```python
from build123d import *

# Parameters (mm, degrees)
F1_DEPTH = 36
F2_R     = 15
F3_T     = -2.5
F4_W     = 67
F4_H     = 27
F5_DEPTH = 3
F6_DEPTH = 100
F7_DEPTH = 5


with BuildPart() as f1:
    # F0 (on Right) → F1 (new body, symmetric)
    with BuildSketch(Plane.YZ):
        Polygon((-28, 0), (0, 0), (0, 32), (-60, 32), (-60, 0), (-60, -28), (-28, -28), align=None)
    extrude(amount=F1_DEPTH, both=True)

    # F2
    f2_edges = [f1.edges().sort_by_distance(p)[0] for p in [
        (0, -60, 32),
        (0, -28, 0),
    ]]
    fillet(f2_edges, radius=F2_R)

    # F3
    f3_openings = [f1.faces().sort_by_distance(p)[0] for p in [
        (0, 0, 16),
    ]]
    offset(amount=F3_T, openings=f3_openings)

    # F4 (on face) → F5 (cut)
    with BuildSketch(Plane(origin=(0, 0, -28), x_dir=(1, 0, 0), z_dir=(0, 0, -1))):
        with Locations((0, 44)):
            Rectangle(F4_W, F4_H)
    extrude(amount=-F5_DEPTH, mode=Mode.SUBTRACT)

    # F6 (add): a face of the model
    f6_faces = [f1.faces().sort_by_distance(p)[0] for p in [
        (-35.2120913759, -44, -28),
    ]]
    extrude(f6_faces, amount=F6_DEPTH)

    # F7 (add): a face of the model
    f7_faces = [f1.faces().sort_by_distance(p)[0] for p in [
        (0, 0, 0.7879086241),
    ]]
    extrude(f7_faces, amount=F7_DEPTH)


solid = f1.part
```
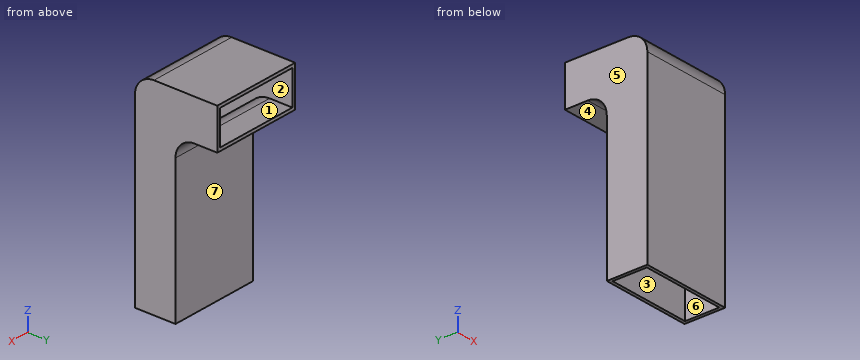
Input: part model. Units: mm. Frame: model coordinates. Face numbers are marked on the shaded views. A direction names the side the tool comes from. Give positions to 0.01 mm unless a question says otherwise; leave off trailing zeros. Loops run counter-clockwise (first coordinate to the right, second up) from the corner with the lowest first, then second, coordinate; pieces in that order, holes last. Notation, with made-up numbers: (36.5, 13.5) -> (67.5, 13.5) arc R8 ccw to (67.5, 20.5) -> close; hole circle Ø8 at (42, 43.5). An arc over 180 degrees is marked (long way). Use a Markdown table: item, result.
Q1. Section query B-B, the plane z = -20. Return the cut outline in (x, y), plus the area to 3 significant figures.
Entries:
| item | result |
|---|---|
| outline | (-36, -60) -> (36, -60) -> (36, -28) -> (-36, -28) -> close; hole (-33.5, -57.5) -> (33.5, -57.5) -> (33.5, -30.5) -> (-33.5, -30.5) -> close |
| area | 495 mm² |
Q2. Section query A-A, the plane x = -20. Return the cut outline in (y, z).
Entries:
| item | result |
|---|---|
| outline | (-60, -128) -> (-57.5, -128) -> (-57.5, 17) arc R12.5 cw to (-45, 29.5) -> (5, 29.5) -> (5, 32) -> (-45, 32) arc R15 ccw to (-60, 17) -> close; (-30.5, -128) -> (-28, -128) -> (-28, -15) arc R15 cw to (-13, 0) -> (5, 0) -> (5, 2.5) -> (-13, 2.5) arc R17.5 ccw to (-30.5, -15) -> close |
Q3. Section query D-D, the plane y = -41.5. Return the cut outline in (x, z), plus the area to 4 significant figures.
Entries:
| item | result |
|---|---|
| outline | (-36, -128) -> (-33.5, -128) -> (-33.5, 29.5) -> (33.5, 29.5) -> (33.5, -128) -> (36, -128) -> (36, 32) -> (-36, 32) -> close |
| area | 967.5 mm² |
Q4. Ray query, probe 1 along Z at (x, y) = (-18, -11.5); probe 2 along X at (y, z) = (-13, 21); probe 3 along Y at (x, z) = (14, -92.5). Return the intervals inside material, ascending. Write a range as from..to.
Entries:
| item | result |
|---|---|
| probe 1 | z = 0..2.5, 29.5..32 |
| probe 2 | x = -36..-33.5, 33.5..36 |
| probe 3 | y = -60..-57.5, -30.5..-28 |
Q5. First-contact query: P1, Ø12, axis at x = 12, z = -41.5, coming from the +Y side; P2, Ø9, axis at x = -9.5, y = -2.5, coming from the -Z side; P3, Ø8, axis at x = -26, z = -14.5, coming from the +Y side. Flat tips, straight axial feed; report the tip coordinate or a pass-through.
Entries:
| item | result |
|---|---|
| P1 | stops at y = -28 |
| P2 | stops at z = 0 |
| P3 | stops at y = -27.31 |
Q6. Section query C-C, the plane y = -1.5. Return the cut outline in (x, z).
Entries:
| item | result |
|---|---|
| outline | (-36, 0) -> (36, 0) -> (36, 32) -> (-36, 32) -> close; hole (-33.5, 2.5) -> (33.5, 2.5) -> (33.5, 29.5) -> (-33.5, 29.5) -> close |
Q7. Pull-direction query (X, two-part tool) for the marked faces 5, 6 and 7; classes: pulls with the +X half, pulls with the -X half, needs draft (parallel to the pull), parting line crosses it, or undercut.
Entries:
| item | result |
|---|---|
| face 5 | pulls with the -X half |
| face 6 | undercut |
| face 7 | needs draft |
Q8. Access query for the marked faces 1, 2, 3 and 4. Directions: +Z, -Z, +X, -X, +Y, -Y. A direction counts if a zero-diameter tool reaches every point of the face in a straight line with its end or side. Return the directions, or none.
Entries:
| item | result |
|---|---|
| face 1 | +Y |
| face 2 | none |
| face 3 | -Z |
| face 4 | -Z, +X, -X, +Y |
